Geometry: final body of the model. Coordinates: model frame, mm. Face numbers are marked on the shaded views. Coordinates: 2 decimals unless noted, no trailing zeros. Loops run counter-clockwise (first coordinate to the right, second up) from the corner with the lowest first, then second, coordinate; pieces in that order, holes last. Notation, with made-up numbers: (-34.75, 34.25) - (5.25, 34.25) arc R24 ccw to (5.25, 63.25) - close; hole circle Ø3 at (9.5, 17.25). An arc over 180 degrees is marked (long way). Put each result on its own line as item: value. Start each with the question number.
1) Contact query for flat-ended pins moving along their axis: pin 1 Ø4 at (y, z) = (302, 53) entering from -X; pin 2 Ø18 at (x, y) = (-364.14, -364.14) entering from -Z; pin 3 Ø5 at (y, z) = (431, 26) entering from -X; pin 4 Ø2 at (x, z) = (-211.5, 9) entering from +Y. Output: stop coordinate, or through.
2) Section A-A on y = 0. Output: boundary loops of the cut face in (x, z) (3 decimals), and give its area (3 significant figures).
3) Section D-D on y = 439. Output: boundary loops of the cut face in (x, z), and give its area (3 significant figures).
4) Material intervals for line 1 along Y through (x, z) = (0, 41) (3 decimals); line 2 along X through (y, z) = (-366, 11); line 3 along X through (y, z) = (207.5, 10), sorted ascending. Write a range as from..to.
5) Draft query along X for the marked faces 1, 2 and 3. Return one class per face: +X half, -X half, draft (parallel to the pull), parting line (faces both ways), or undercut.
6) Section C-C on x = -232.5. Output: boundary loops of the cut face in (y, z).
```python
from build123d import *

# Parameters (mm, degrees)
SKETCH1_R               = 564.965
SKETCH1_R_2             = 464.965
BOSS_EXTRUDE1_DEPTH     = 70
CUT_EXTRUDE2_DEPTH      = 803.041708672
CUT_EXTRUDE2_DEPTH_BACK = 803.041708672
SKETCH3_R               = 15


with BuildPart() as part:
    # Sketch1 → Boss-Extrude1 (new body)
    with BuildSketch(Plane.XY):
        Circle(SKETCH1_R)
        Circle(SKETCH1_R_2, mode=Mode.SUBTRACT)
    extrude(amount=BOSS_EXTRUDE1_DEPTH)

    # Sketch3 → Cut-Extrude2 (cut, two sides: drawn at the far end of the back side and taken through both)
    with BuildSketch(Plane.XY.offset(70).offset(-CUT_EXTRUDE2_DEPTH_BACK)):
        with Locations((197.068573748, 475.76562346)):
            Circle(SKETCH3_R)
        with Locations((364.135243574, 364.135243574)):
            Circle(SKETCH3_R)
        with Locations((475.76562346, 197.068573748)):
            Circle(SKETCH3_R)
        with Locations((514.965, 0)):
            Circle(SKETCH3_R)
        with Locations((475.76562346, -197.068573748)):
            Circle(SKETCH3_R)
        with Locations((364.135243574, -364.135243574)):
            Circle(SKETCH3_R)
        with Locations((197.068573748, -475.76562346)):
            Circle(SKETCH3_R)
        with Locations((0, -514.965)):
            Circle(SKETCH3_R)
        with Locations((-197.068573748, -475.76562346)):
            Circle(SKETCH3_R)
        with Locations((-364.135243574, -364.135243574)):
            Circle(SKETCH3_R)
        with Locations((-475.76562346, -197.068573748)):
            Circle(SKETCH3_R)
        with Locations((-514.965, 0)):
            Circle(SKETCH3_R)
        with Locations((-475.76562346, 197.068573748)):
            Circle(SKETCH3_R)
        with Locations((-364.135243574, 364.135243574)):
            Circle(SKETCH3_R)
        with Locations((-197.068573748, 475.76562346)):
            Circle(SKETCH3_R)
        with Locations((0, 514.965)):
            Circle(SKETCH3_R)
    extrude(amount=CUT_EXTRUDE2_DEPTH + CUT_EXTRUDE2_DEPTH_BACK, mode=Mode.SUBTRACT)


solid = part.part
```
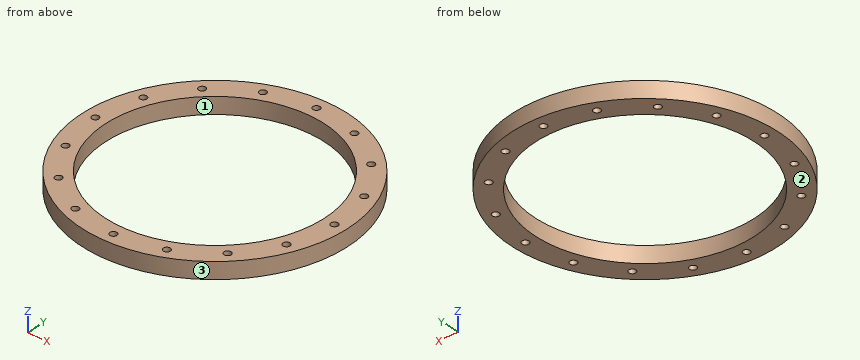
Answer block:
1. pin 1: stops at x = -478.73
1. pin 2: passes through
1. pin 3: stops at x = -368.2
1. pin 4: stops at y = 524.29
2. outline: (-564.965, 0) - (-529.965, 0) - (-529.965, 70) - (-564.965, 70) - close; (-499.965, 0) - (-464.965, 0) - (-464.965, 70) - (-499.965, 70) - close; (464.965, 0) - (499.965, 0) - (499.965, 70) - (464.965, 70) - close; (529.965, 0) - (564.965, 0) - (564.965, 70) - (529.965, 70) - close
2. area: 9,800 mm²
3. outline: (-355.62, 0) - (-153.2, 0) - (-153.2, 70) - (-355.62, 70) - close; (153.2, 0) - (355.62, 0) - (355.62, 70) - (153.2, 70) - close
3. area: 28,300 mm²
4. line 1: y = -564.965..-529.965, -499.965..-464.965, 464.965..499.965, 529.965..564.965
4. line 2: x = -430.38..-379.02, -349.25..-286.77, 286.77..349.25, 379.02..430.38
4. line 3: x = -525.48..-486.54, -464.99..-416.1, 416.1..464.99, 486.54..525.48
5. face 1: undercut
5. face 2: draft
5. face 3: parting line
6. outline: (-514.91, 0) - (-402.66, 0) - (-402.66, 70) - (-514.91, 70) - close; (402.66, 0) - (514.91, 0) - (514.91, 70) - (402.66, 70) - close
